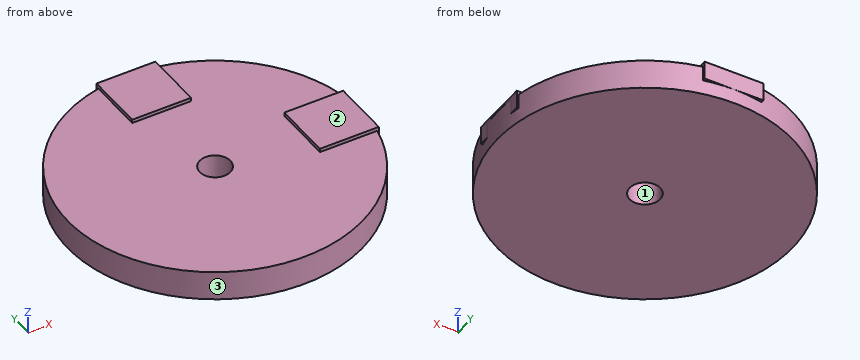
```python
from build123d import *

# Parameters (mm, degrees)
F0_R     = 7.9375
F0_R_2   = 0.8255
F1_DEPTH = 0.79375
F2_W     = 3.175
F2_H     = 3.175
F3_DEPTH = 0.9871898219
F4_W     = 3.175
F4_H     = 3.175
F5_DEPTH = 0.987298


with BuildPart() as f1:
    # F0 (on Top) → F1 (new body, symmetric)
    with BuildSketch(Plane.XY):
        Circle(F0_R)
        Circle(F0_R_2, mode=Mode.SUBTRACT)
    extrude(amount=F1_DEPTH, both=True)

    # F2 (on Top) → F3 (join)
    with BuildSketch(Plane.XY):
        with Locations((0, 6.35)):
            Rectangle(F2_W, F2_H)
    extrude(amount=F3_DEPTH)

    # F4 (on Top) → F5 (join)
    with BuildSketch(Plane.XY):
        with Locations((6.2804043693, 0)):
            Rectangle(F4_W, F4_H)
    extrude(amount=F5_DEPTH)


solid = f1.part
```
Work out the finished part from the listing and answer in its coordinate system (mm). Face numbers are marked on the shaded views. Coordinates: 2 decimals unless noted, no trailing zeros. Loops run counter-clockwise (first coordinate to the right, second up) from the corner with the lowest first, then second, coordinate; pieces in that order, holes last. Notation, with made-up numbers: M -30,14.5 L 7,14.5 A29 ccw 7,36.5 Z; hole C -19,-1.5 d11. An arc over 180 degrees is marked long. Use CSV: the item, a comma, the result in double quotes. Start each with the question number.
(1) Find section D-D, the plane x = 5.25. Give the vertices of the cut face in (y, z).
(2) Consider line 1 (Y direction, x = 0, z = 0.35); line 2 (Z direction, x = -3.5, y = 0.5); line 3 (Y direction, x = 3.75, z = -0.2). Determine where each line is inside the solid, lowest interval first.
(3) Find section B-B, the plane y = 0. Give the vertices of the cut face in (x, z).
(4) Given pin 1 Ø0.5 at (x, z) = (6, 0.5) entering from +Y; pin 2 Ø0.8 at (y, z) = (7, 0.5) entering from +X; pin 3 Ø1.3 at (x, y) = (0, 0) entering from -Z; pin 4 Ø0.8 at (y, z) = (-0.5, 0.5) entering from +X, each flat-ended and moving along its own axis, determine where each tip first touches the part or whether it passes through.
(5) Find section C-C, the plane y = 6.5. Give the vertices of the cut face in (x, z).
(6) For a pull along X with two mould halves and no side action, classify the marked faces 1, 2 and 3 as +X half, -X half, draft (parallel to the pull), parting line (faces both ways), or undercut.
Recorded:
1,outline,"M -5.95,-0.79 L 5.95,-0.79 L 5.95,0.79 L 1.59,0.79 L 1.59,0.99 L -1.59,0.99 L -1.59,0.79 L -5.95,0.79 Z"
2,line 1,"y = -7.94 to -0.83, 0.83 to 7.94"
2,line 2,"z = -0.79 to 0.79"
2,line 3,"y = -7 to 7"
3,outline,"M -7.94,-0.79 L -0.83,-0.79 L -0.83,0.79 L -7.94,0.79 Z; M 0.83,-0.79 L 7.94,-0.79 L 7.94,0.79 L 7.87,0.79 L 7.87,0.99 L 4.69,0.99 L 4.69,0.79 L 0.83,0.79 Z"
4,pin 1,"stops at y = 5.47"
4,pin 2,"stops at x = 4.41"
4,pin 3,"passes through"
4,pin 4,"stops at x = 7.94"
5,outline,"M -4.56,-0.79 L 4.56,-0.79 L 4.56,0.79 L 1.59,0.79 L 1.59,0.99 L -1.59,0.99 L -1.59,0.79 L -4.56,0.79 Z"
6,face 1,"undercut"
6,face 2,"draft"
6,face 3,"parting line"
